Build history of the part. All positions in model axes, mm. A direction names the side the tool comes from. Give positions to 0.01 mm unless a question says otherwise; leave off trailing zeros. Write each loop counter-clockwise with the first axis right and the second up, starting at its lowest first coordinate (ties: lowest second). Pieces come first, ordered by that corner, then holes. Notation, with made-up numbers: (-2, 78) -> (53, 78) arc R6 ccw to (53, 82) -> close; hole circle Ø6 at (-9.5, 89.25). An arc over 180 degrees is marked (long way). Write item = value, one per line. Start each with the question number.
Q1. Saw through at B-B, the plane y = -39. List the corners of the cut face in (x, z), then the cut area to 3 significant figures.
Q2. Saw through at A-A, the plane z = 5.25. List the corners of the cut face in (x, y), then the cut area to 3 significant figures.
Q3. Mould opens along X. For faces 1 (the face through (-29, 35, 7.5)), 2 (the face through (40, -1, 4)), 3 (the face through (-23, 0, 7.5)) say: pulls with the +X half, pulls with the -X half, needs draft (parallel to the pull), parting line crosses it, or undercut.
Q4. Tool access for faces 4 (the face through (-11.07, 19.47, 16.13)), 5 (the face through (-40, 1, 4)): list every direction of +Z, -Z, +X, -X, +Y, -Y with a clear straight run to the whole face (end or side of a thin tool).
Q5. Drop flat-ended pins along their axis: P1, Ø6, axis at x = 1.5, y = -34, coming from the +Z side; P2, Ø22, axis at x = -26.5, y = -4, coming from the +Z side; P3, Ø5, axis at x = -14.5, z = 19.5, coming from the -Y side; P4, Ø5, axis at y = -24.5, z = 22.5, coming from the +X side. Give the stop position or say it passes through.
Q6. Saw through at C-C, the plane z = 22.5. List the corners of the cut face in (x, y), then the cut area to 3 significant figures.
Q7. Wall check: line 1 (Y direction, x = 0, z = 20.5); line 2 (Y direction, x = -25, z = 6.25); line 3 (X direction, y = 9, z = 15.5). Give the ranges that are in metal, low to high.
Autodesk Inventor part; units mm, degrees
ref_plane "YZ Plane" through (0, 0, 0) normal (1, 0, 0) x (0, 1, 0)
ref_plane "XZ Plane" through (0, 0, 0) normal (0, 1, 0) x (-1, 0, 0)
ref_plane "XY Plane" through (0, 0, 0) normal (0, 0, 1) x (1, 0, 0)
sketch "Sketch1" plane through (0, 0, 0) normal (0, 0, 1) x (1, 0, 0)
  line L0 (-25, -56.5) -> (25, -56.5)
  line L1 (40, -41.5) -> (40, 41.5)
  line L2 (25, 56.5) -> (-25, 56.5)
  line L3 (-40, 41.5) -> (-40, -41.5)
  arc A0 (40, 41.5) -> (25, 56.5) centre (25, 41.5) ccw
  arc A1 (25, -56.5) -> (40, -41.5) centre (25, -41.5) ccw
  arc A2 (-40, -41.5) -> (-25, -56.5) centre (-25, -41.5) ccw
  arc A3 (-25, 56.5) -> (-40, 41.5) centre (-25, 41.5) ccw
  circle A4 centre (25, 41.5) radius 5
  circle A5 centre (25, -41.5) radius 5
  circle A6 centre (-25, -41.5) radius 5
  circle A7 centre (-25, 41.5) radius 5
  point P0 (0, 0)
  point P1 (0, 56.5)
  point P2 (40, 0)
  dimension "d0" = 113
  dimension "d1" = 80
  dimension "d2" = 15
  dimension "d3" = 10
extrude "Extrusion1" add sketch "Sketch1" along normal blind 7.5
sketch "Sketch2" plane through (0, 0, 7.5) normal (0, 0, 1) x (1, 0, 0)
  line L0 (40, -41.5) -> (40, 41.5)
  line L1 (25, 56.5) -> (-25, 56.5)
  circle A0 centre (0, 39) radius 10
  arc A1 (14.2128, 34.2045) -> (-14.2128, 34.2045) centre (0, 39) ccw
  arc A2 (14.2128, 34.2045) -> (25.4628, 14.7045) centre (28.4256, 29.409) ccw
  arc A3 (25.4628, -14.7045) -> (25.4628, 14.7045) centre (22.5, 0) ccw
  circle A4 centre (22.5, 0) radius 10
  arc A5 (-5.9008, 25.2094) -> (5.9008, 25.2094) centre (0, 39) ccw
  arc A6 (9.2778, 23.633) -> (13.8407, 15.7238) centre (28.4256, 29.409) ccw
  arc A7 (13.5151, 12.0113) -> (13.5151, -12.0113) centre (22.5, 0) ccw
  arc A8 (9.2778, 23.633) -> (5.9008, 25.2094) centre (6.8843, 22.911) ccw
  arc A9 (13.5151, 12.0113) -> (13.8407, 15.7238) centre (12.0176, 14.0132) ccw
  arc A10 (-5.9008, 25.2094) -> (-9.2778, 23.633) centre (-6.8843, 22.911) ccw
  arc A11 (25.4628, -14.7045) -> (14.2128, -34.2045) centre (28.4256, -29.409) ccw
  arc A12 (-14.2128, -34.2045) -> (14.2128, -34.2045) centre (0, -39) ccw
  circle A13 centre (0, -39) radius 10
  arc A14 (-14.2128, -34.2045) -> (-25.4628, -14.7045) centre (-28.4256, -29.409) ccw
  arc A15 (-25.4628, 14.7045) -> (-25.4628, -14.7045) centre (-22.5, 0) ccw
  circle A16 centre (-22.5, 0) radius 10
  arc A17 (-25.4628, 14.7045) -> (-14.2128, 34.2045) centre (-28.4256, 29.409) ccw
  arc A18 (13.8407, -15.7238) -> (13.5151, -12.0113) centre (12.0176, -14.0132) ccw
  arc A19 (13.8407, -15.7238) -> (9.2778, -23.633) centre (28.4256, -29.409) ccw
  arc A20 (5.9008, -25.2094) -> (9.2778, -23.633) centre (6.8843, -22.911) ccw
  arc A21 (-13.8407, 15.7238) -> (-13.5151, 12.0113) centre (-12.0176, 14.0132) ccw
  arc A22 (-13.8407, 15.7238) -> (-9.2778, 23.633) centre (-28.4256, 29.409) ccw
  arc A23 (-13.5151, -12.0113) -> (-13.5151, 12.0113) centre (-22.5, 0) ccw
  arc A24 (-9.2778, -23.633) -> (-13.8407, -15.7238) centre (-28.4256, -29.409) ccw
  arc A25 (-13.5151, -12.0113) -> (-13.8407, -15.7238) centre (-12.0176, -14.0132) ccw
  arc A26 (5.9008, -25.2094) -> (-5.9008, -25.2094) centre (0, -39) ccw
  arc A27 (-9.2778, -23.633) -> (-5.9008, -25.2094) centre (-6.8843, -22.911) ccw
  point P0 (0, 0)
  point P1 (0, 54)
  point P2 (37.5, 0)
  point P3 (0, -54)
  point P4 (-37.5, 0)
  point P5 (0, 0)
  point P6 (9.2778, -23.633)
  dimension "d6" = 20
  dimension "d7" = 15
  dimension "d8" = 2.5
  dimension "d9" = 15
  dimension "d10" = 2.5
  dimension "d11" = 20
  dimension "d12" = 2.5
  dimension "d13" = 5
  dimension "d14" = 5
  dimension "d17" = 360
  dimension "d21" = 360
extrude "Extrusion2" add sketch "Sketch2" along normal blind 17.5
fillet "Fillet1" radius 2.5 8 edges at (37.5, 0, 7.5) (15.4328, -21.9131, 7.5) (0, -54, 7.5) (-15.4328, -21.9131, 7.5) (-37.5, 0, 7.5) (-15.4328, 21.9131, 7.5) (0, 54, 7.5) (15.4328, 21.9131, 7.5)
properties part number "DP807"
Report:
q1.outline = (-40, 0) -> (-29.33, 0) -> (-29.33, 7.5) -> (-40, 7.5) -> close; (-20.67, 0) -> (20.67, 0) -> (20.67, 7.5) -> (17.5, 7.5) arc R2.5 cw to (15, 10) -> (15, 25) -> (10, 25) -> (10, 7.5) -> (-10, 7.5) -> (-10, 25) -> (-15, 25) -> (-15, 10) arc R2.5 cw to (-17.5, 7.5) -> (-20.67, 7.5) -> close; (29.33, 0) -> (40, 0) -> (40, 7.5) -> (29.33, 7.5) -> close
q1.area = 648 mm2
q2.outline = (-40, -41.5) arc R15 ccw to (-25, -56.5) -> (25, -56.5) arc R15 ccw to (40, -41.5) -> (40, 41.5) arc R15 ccw to (25, 56.5) -> (-25, 56.5) arc R15 ccw to (-40, 41.5) -> close; hole circle Ø10 at (-25, -41.5); hole circle Ø10 at (-25, 41.5); hole circle Ø10 at (25, -41.5); hole circle Ø10 at (25, 41.5)
q2.area = 8,530 mm2
q3.face_1 = needs draft
q3.face_2 = pulls with the +X half
q3.face_3 = undercut
q4.face_4 = +Z
q4.face_5 = +Z, -Z, -X, +Y, -Y
q5.P1 = 7.5
q5.P2 = 25
q5.P3 = -48
q5.P4 = 15.38
q6.outline = (-25.46, -14.7) arc R15 cw to (-14.21, -34.2) arc R15 ccw (long way) to (14.21, -34.2) arc R15 cw to (25.46, -14.7) arc R15 ccw to (25.46, 14.7) arc R15 cw to (14.21, 34.2) arc R15 ccw (long way) to (-14.21, 34.2) arc R15 cw to (-25.46, 14.7) arc R15 ccw to start; hole circle Ø20 at (-22.5, 0); hole (-13.84, -15.72) arc R20 cw to (-9.28, -23.63) arc R2.5 ccw to (-5.9, -25.21) arc R15 cw to (5.9, -25.21) arc R2.5 ccw to (9.28, -23.63) arc R20 cw to (13.84, -15.72) arc R2.5 ccw to (13.52, -12.01) arc R15 cw to (13.52, 12.01) arc R2.5 ccw to (13.84, 15.72) arc R20 cw to (9.28, 23.63) arc R2.5 ccw to (5.9, 25.21) arc R15 cw to (-5.9, 25.21) arc R2.5 ccw to (-9.28, 23.63) arc R20 cw to (-13.84, 15.72) arc R2.5 ccw to (-13.52, 12.01) arc R15 cw to (-13.52, -12.01) arc R2.5 ccw to start; hole circle Ø20 at (0, -39); hole circle Ø20 at (0, 39); hole circle Ø20 at (22.5, 0)
q6.area = 1,940 mm2
q7.line_1 = -54 to -49, -29 to -24, 24 to 29, 49 to 54
q7.line_2 = -56.5 to -46.5, -36.5 to 36.5, 46.5 to 56.5
q7.line_3 = -34.5 to -26.86, -18.14 to -10.5, 10.5 to 18.14, 26.86 to 34.5
